from build123d import *

# Parameters (mm, degrees)
SKETCH_1_R      = 1.7
EXTRUDE_1_DEPTH = 2
FILLET_1_R      = 2
SKETCH_3_R      = 8
SKETCH_3_R_2    = 2.5
EXTRUDE_2_DEPTH = 12
SKETCH_5_W      = 8
SKETCH_5_H      = 8
EXTRUDE_3_DEPTH = 12
SKETCH_6_W      = 8
SKETCH_6_H      = 4
EXTRUDE_4_DEPTH = 10


with BuildPart() as part:
    # 草图1 → 凸台-拉伸1 (new body)
    with BuildSketch(Plane(origin=(0, 0, 0), x_dir=(1, 0, 0), z_dir=(0, 1, 0))):
        with BuildLine():
            Line((10, 28.35), (10, 12.064213562))
            Line((10, 12.064213562), (6.642893219, 8.707106781))
            ThreePointArc((6.642893219, 8.707106781), (6.355850084, 8.108009006), (6.507537143, 7.461245571))
            Line((6.507537143, 7.461245571), (10, 2))
            Line((10, 2), (10, 0))
            ThreePointArc((10, 0), (9.22383297, -1.87383297), (7.35, -2.65))
            Line((7.35, -2.65), (-7.35, -2.65))
            ThreePointArc((-7.35, -2.65), (-9.22383297, -1.87383297), (-10, 0))
            Line((-10, 0), (-10, 2))
            Line((-10, 2), (-6.507537143, 7.461245571))
            ThreePointArc((-6.507537143, 7.461245571), (-6.355850084, 8.108009006), (-6.642893219, 8.707106781))
            Line((-6.642893219, 8.707106781), (-10, 12.064213562))
            Line((-10, 12.064213562), (-10, 28.35))
            ThreePointArc((-10, 28.35), (0, 38.35), (10, 28.35))
        make_face()
        with Locations(Location((7.35, 0, 0), (0, 0, 270))):
            Circle(SKETCH_1_R, mode=Mode.SUBTRACT)
        with Locations(Location((-7.35, 0, 0), (0, 0, 90))):
            Circle(SKETCH_1_R, mode=Mode.SUBTRACT)
    extrude(amount=EXTRUDE_1_DEPTH)

    # 圆角1
    fillet_1_edges = [part.edges().sort_by_distance(p)[0] for p in [
        (-10, 1, -2),
        (-10, 1, -12.064213562),
        (10, 1, -12.064213562),
        (10, 1, -2),
    ]]
    fillet(fillet_1_edges, radius=FILLET_1_R)

    # 草图3 → 凸台-拉伸2 (add)
    with BuildSketch(Plane(origin=(0, 2, 0), x_dir=(1, 0, 0), z_dir=(0, 1, 0))):
        with Locations(Location((0, 28.35, 0), (0, 0, 90))):
            Circle(SKETCH_3_R)
        with Locations(Location((0, 17.35, 0), (0, 0, 90))):
            Circle(SKETCH_3_R_2)
    extrude(amount=EXTRUDE_2_DEPTH)

    # 草图4 → 旋转1 (revolve)
    with BuildSketch(Plane(origin=(0, 14, 0), x_dir=(1, 0, 0), z_dir=(0, 1, 0))):
        with BuildLine():
            Line((0, 34.35), (0, 22.35))
            ThreePointArc((0, 22.35), (6, 28.35), (0, 34.35))
        make_face()
    revolve(axis=Axis((0, 14, -36.05355047), (0, 0, 1)))

    # 草图5 → 凸台-拉伸3 (add)
    with BuildSketch(Plane.XZ):
        with Locations((-0.398314742, -17.513469077)):
            Rectangle(SKETCH_5_W, SKETCH_5_H)
    extrude(amount=EXTRUDE_3_DEPTH)

    # 草图6 → 凸台-拉伸4 (add)
    with BuildSketch(Plane.XZ):
        with Locations((0, 0.65)):
            Rectangle(SKETCH_6_W, SKETCH_6_H)
    extrude(amount=EXTRUDE_4_DEPTH)


solid = part.part
For this review, take the finished solid that the model builds, in its own axes (mm). A direction names the side the tool comes from. Round coordinates to 2 decimals unless told otherwise and drop trailing zeros. Order: outer loops, then holes, each group sorted by start corner. A loop starts at its lowest first (then second) coordinate and runs counter-clockwise, first axis right, second up. Notation, with made-up numbers: M 80,30.25 L 133,30.25 A20 cw 133,49.25 Z; hole C 63.25,-11.75 d1. An arc over 180 degrees is marked long. Use a Markdown table: item, result. Add a question column.
Item 1: Tool access review of faces 4 (the flat face through (3.602, -6, -18)), 5 (the flat face through (0, -6, -13.513)), 6 (the flat face through (4, -5, 1)), 7 (the flat face through (-8.009, 0.986, -10.073)): name each direction out of +Z, -Z, +X, -X, +Y, -Y from which nothing blocks a thin tool from reaching the whole face with its end or side.
Item 2: Add section D-D, the plane z = -31.5. Give the boundary of the cut face in (x, y), then the cut area to 3 significant figures.
Item 3: Insertion check: pin 1 (1.2 mm diameter, centred on y = -4.5, z = 1.5, fed in from +X); pin 2 (8 mm diameter, centred on x = 1, y = 14, fed in from +Z); pin 3 (1.2 mm diameter, centred on x = 1, z = 1, fed in from -Y); pin 4 (5 mm diameter, centred on y = -3, z = -7.5, fed in from -X). Each pin has a flat end and moves straight along its axis. Give the tip position at first contact, or say it passes through.
Item 4: Mouldability with a two-part tool opening along X and no side actions: class faces 1 (the cylindrical face through (-0.22, 0.986, -38.348)), 2 (the cylindrical face through (9.92, 1.01, -1.98)), 3 (the cylindrical face through (9.036, 0.986, -0.221)) as released by +X, released by -X, zero draft, split by the parting line, or undercut.
Item 5: Add section A-A, the plane y = -0.5. Give the boundary of the cut face in (x, z).
Item 6: To check wall thickness, follow line 1 along Z through (x, y) = (1, -0.5); line 2 along Z through (x, y) = (-7.35, 0.9); line 3 along Y through (x, z) = (5, -1). State the ranges of each line that lie inside material, in increasing order.
Item 7: Add section B-B, the plane z = -17.35. Give the boundary of the cut face in (x, y).
Item 8: Add section C-C, the plane x = 4.5. Give the boundary of the cut face in (y, z), then the cut area to 3 significant figures.
Geometry results:
| question | item | result |
|---|---|---|
| 1 | face 4 | -Z, +X, -Y |
| 1 | face 5 | +X, -X, -Y |
| 1 | face 6 | +Z, -Z, +X, -Y |
| 1 | face 7 | -X, +Y, -Y |
| 2 | outline | M -9.49,0 L 9.49,0 L 9.49,2 L 7.35,2 L 7.35,14 L 5.11,14 A5.11 ccw -5.11,14 L -7.35,14 L -7.35,2 L -9.49,2 Z |
| 2 | area | 255 mm² |
| 3 | pin 1 | stops at x = 4 |
| 3 | pin 2 | stops at z = -14.85 |
| 3 | pin 3 | stops at y = -10 |
| 3 | pin 4 | passes through |
| 4 | face 1 | split by the parting line |
| 4 | face 2 | released by +X |
| 4 | face 3 | undercut |
| 5 | outline | M -4.4,-21.51 L 3.6,-21.51 L 3.6,-13.51 L -4.4,-13.51 Z; M -4,-1.35 L 4,-1.35 L 4,2.65 L -4,2.65 Z |
| 6 | line 1 | z = -21.51 to -13.51, -1.35 to 2.65 |
| 6 | line 2 | z = -35.13 to -9.41, -6.14 to -1.7, 1.7 to 2.65 |
| 6 | line 3 | y = 0 to 2 |
| 7 | outline | M -10,0 L -4.4,0 L -4.4,-12 L 3.6,-12 L 3.6,0 L 10,0 L 10,2 L 2.5,2 L 2.5,14 L -2.5,14 L -2.5,2 L -10,2 Z |
| 8 | outline | M 0,-37.28 L 2,-37.28 L 2,-34.96 L 14,-34.96 L 14,-32.32 A3.97 ccw 14,-24.38 L 14,-21.74 L 2,-21.74 L 2,2.65 L 0,2.65 Z |
| 8 | area | 263 mm² |
